Autodesk Inventor part; units mm, degrees
ref_plane "YZ Plane" through (0, 0, 0) normal (1, 0, 0) x (0, 1, 0)
ref_plane "XZ Plane" through (0, 0, 0) normal (0, 1, 0) x (-1, 0, 0)
ref_plane "XY Plane" through (0, 0, 0) normal (0, 0, 1) x (1, 0, 0)
sketch "Sketch1" plane through (0, 0, 0) normal (0, 1, 0) x (-1, 0, 0)
  circle A0 centre (0, 0) radius 36
  circle A1 centre (0, 0) radius 15
  dimension "d0" = 72
  dimension "d1" = 30
extrude "Extrusion1" add sketch "Sketch1" along normal blind 5
sketch "Sketch2" plane through (0, 0, 0) normal (0, -1, 0) x (1, 0, 0)
  circle A0 centre (0, 0) radius 36
  circle A1 centre (0, 0) radius 15
  circle A2 centre (0, 0) radius 20.05
  dimension "d4" = 40.1
extrude "Extrusion2" add sketch "Sketch2" along normal blind 11.5 contours A2
sketch "Sketch3" plane through (0, -11.5, 0) normal (0, -1, 0) x (1, 0, 0)
  circle A0 centre (0, 0) radius 7.5
  circle A1 centre (0, 0) radius 20.05
  circle A2 centre (0, 0) radius 15
  circle A3 centre (0, 0) radius 6.5
  dimension "d7" = 15
  dimension "d8" = 13
extrude "Extrusion3" add sketch "Sketch3" along normal blind 29.5 and the other way blind 8.5 contours A0
extrude "Extrusion4" add sketch "Sketch3" against normal up to surface (8.5 mm away) contours A2
sketch "Sketch4" plane through (0, -41, 0) normal (0, -1, 0) x (1, 0, 0)
  circle A0 centre (0, 0) radius 7.5
  circle A1 centre (0, 0) radius 6.5
  circle A2 centre (0, 0) radius 8.45
  dimension "d15" = 16.9
extrude "Extrusion5" add sketch "Sketch4" against normal blind 5 contours A2
sketch "Sketch5" plane through (0, -36, 0) normal (0, 1, 0) x (1, 0, 0)
  point P0 (0, 0)
sketch "Sketch6" plane through (0, 0, 0) normal (0, 0, 1) x (1, 0, 0)
  line L0 (8.45, -36) -> (-8.45, -36)
  line L1 (-8.45, -41) -> (8.45, -41)
  line L2 (8.45, -32) -> (-8.45, -32)
  line L3 (-8.45, -32) -> (-8.45, -22)
  line L4 (-8.45, -22) -> (8.45, -22)
  line L5 (8.45, -22) -> (8.45, -32)
  point P0 (0, 0)
  dimension "d18" = 10
  dimension "d21" = 9
extrude "Extrusion6" add sketch "Sketch6" along normal mid plane 20
properties part number "Axis1_bottom"
Build history of the part. All positions in model axes, mm. A direction names the side the tool comes from. Coordinates: 2 decimals unless noted, no trailing zeros. Write each loop counter-clockwise with the first axis right and the second up, starting at its lowest first coordinate (ties: lowest second). Pieces come first, ordered by that corner, then holes.
(1) Drill centre lines: line 1 (Y direction, x = -8, z = 2); line 2 (X direction, y = -35.25, z = 0). Where is each one in solid material? Low to high.
(2) Cut at B-B on z = -11.5. List the corners of the cut face in (x, y).
(3) 3-axis set-ups, long thin cutter, end or side, ignore diameter. For faces 5 (the flat face through (3, -3, -6)), 6 (the cylindrical face through (-5.158, -36.437, 3.955)), 7 (the flat face through (8, -32, 0)): which of +Z, -Z, +X, -X, +Y, -Y reach the whole face in a straight line?
(4) Cut at D-D on y = -24.5. List the corners of the cut face in (x, z), and give its area (3 significant figures).
(5) Pin check, flat tips, straight feed: pin 1 Ø8 at (x, z) = (0, 0) entering from -Y; pin 2 Ø3 at (y, z) = (-29, -2) entering from -X; pin 3 Ø18 at (x, z) = (0, 0) entering from +Y. Stop position of each tip, or through.
(6) Cut at C-C on x = -9.5. List the corners of the cut face in (y, z).
(7) Cut at A-A on y = -38. List the corners of the cut face in (x, z).
(8) Mould opens along Y. For faces 1 (the cylindrical face through (-7.493, -16.676, -0.33)), 2 (the flat face through (0, -32, 0)), 3 (the flat face through (0, -27, 10)), 4 (the flat face through (-8, -22, 0)) say: pulls with the +Y half, pulls with the -Y half, needs draft (parallel to the pull), parting line crosses it, or undercut.
Working result:
1. line 1: y = -41 to -36, -32 to -22, -11.5 to -3
1. line 2: x = -7.5 to -6.5, 6.5 to 7.5
2. outline: (-34.11, 0) - (-16.42, 0) - (-16.42, -11.5) - (16.42, -11.5) - (16.42, 0) - (34.11, 0) - (34.11, 5) - (9.63, 5) - (9.63, -3) - (-9.63, -3) - (-9.63, 5) - (-34.11, 5) - close
3. face 5: +Y
3. face 6: -Y
3. face 7: none
4. outline: (-8.45, -10) - (8.45, -10) - (8.45, 10) - (-8.45, 10) - close
4. area: 338 mm2
5. pin 1: stops at y = -32
5. pin 2: stops at x = -8.45
5. pin 3: stops at y = -3
6. outline: (-11.5, -17.66) - (0, -17.66) - (0, -34.72) - (5, -34.72) - (5, -11.61) - (-3, -11.61) - (-3, 11.61) - (5, 11.61) - (5, 34.72) - (0, 34.72) - (0, 17.66) - (-11.5, 17.66) - close
7. outline: circle Ø16.9 at (0, 0); hole circle Ø13 at (0, 0)
8. face 1: undercut
8. face 2: pulls with the -Y half
8. face 3: needs draft
8. face 4: undercut
